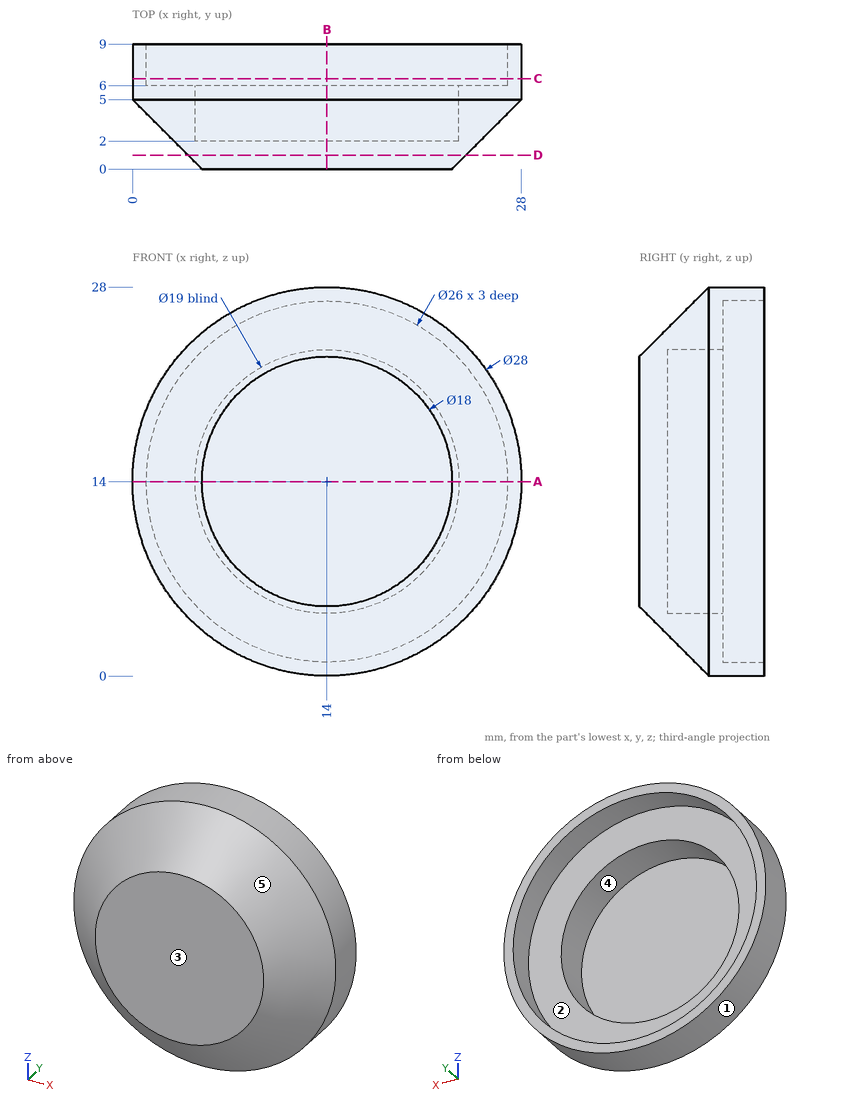
Here's the drawing with two shaded views (mm, measured from the low corner). I have some questions. A direction names the side the tool comes from. Coordinates: 2 decimals unless noted, no trailing zeros. Order: outer loops, then holes, each group sorted by start corner. A loop starts at its lowest first (then second) coordinate and runs counter-clockwise, first axis right, second up.
Q1. Suppose I cut it at C-C on y = 6.5. Please give me the cut outline in (x, z).
Q2. Suppose I cut it at A-A on z = 14. Please give me the cut outline in (x, y), and give its area (3 significant figures).
Q3. Please list where these lines run through material, in increasing order: L1, parallel to X at y = 7.7, z = 14; L2, parallel to X at y = 3.2, z = 14; L3, parallel to Z at x = 8.75, y = 7.
Q4. Will these pins go through, and if not, where does the flat tip stop? pin 1 (1 mm diameter, centred on x = 9, z = 4.5, fed in from -Y); pin 2 (2 mm diameter, centred on y = 1.5, z = 13, fed in from +X); pin 3 (1 mm diameter, centred on x = 3, z = 15.5, fed in from -Y).
Q5. Suppose I cut it at B-B on x = 14. Please give me the cut outline in (y, z), and give its area (3 significant figures).
Q6. Thinking about a two-plate mould opening in Z: for the marked faces 1, 2 and 3, which applies, released by +Z, released by -Z, zero draft, split by the parting line, or undercut?
Q7. Suppose I cut it at D-D on y = 1. Please give me the cut outline in (x, z).
Q8. Which directions (+Z, -Z, +X, -X, +Y, -Y) give clear straight access to the entire face, cutting with the end or side of a thin tool? Please do the marked faces 4 and 5.
Answer:
1. outline: circle Ø28 at (14, 14); hole circle Ø26 at (14, 14)
2. outline: (0, 5) - (5, 0) - (23, 0) - (28, 5) - (28, 9) - (27, 9) - (27, 6) - (23.5, 6) - (23.5, 2) - (4.5, 2) - (4.5, 6) - (1, 6) - (1, 9) - (0, 9) - close
2. area: 73.0 mm2
3. L1: x = 0 to 1, 27 to 28
3. L2: x = 1.8 to 4.5, 23.5 to 26.2
3. L3: z = 1.02 to 2.11, 25.89 to 26.98
4. pin 1: stops at y = 1.24
4. pin 2: stops at x = 25.46
4. pin 3: stops at y = 1.6
5. outline: (0, 5) - (5, 0) - (9, 0) - (9, 1) - (6, 1) - (6, 4.5) - (2, 4.5) - (2, 23.5) - (6, 23.5) - (6, 27) - (9, 27) - (9, 28) - (5, 28) - (0, 23) - close
5. area: 73.0 mm2
6. face 1: split by the parting line
6. face 2: undercut
6. face 3: zero draft
7. outline: circle Ø20 at (14, 14)
8. face 4: +Y
8. face 5: -Y
